Autodesk Inventor part; units mm, degrees
ref_plane "YZ Plane" through (0, 0, 0) normal (1, 0, 0) x (0, 1, 0)
ref_plane "XZ Plane" through (0, 0, 0) normal (0, 1, 0) x (-1, 0, 0)
ref_plane "XY Plane" through (0, 0, 0) normal (0, 0, 1) x (1, 0, 0)
sketch "Boceto1" plane through (0, 0, 0) normal (0, 1, 0) x (-1, 0, 0)
  circle A0 centre (0, 0) radius 19.6
  dimension "d0" = 39.2
extrude "Extrusión1" add sketch "Boceto1" along normal blind 60
sketch "Boceto2" plane through (0, 60, 0) normal (0, 1, 0) x (1, 0, 0)
  circle A0 centre (0, 0) radius 19.6
hole "Agujero1" at (0, 60, 0) direction (0, -1, 0) diameter 35 depth 20 tip angle 118
sketch "Boceto3" plane through (0, 0, 0) normal (0, -1, 0) x (1, 0, 0)
  circle A0 centre (0, 0) radius 19.6
hole "Agujero2" at (0, 0, 0) direction (0, 1, 0) diameter 10 depth 20 tip angle 118
thread "Rosca1"
fillet "Empalme1" radius 10 1 edges at (19.6, 0, 0)
properties part number "Casquillo"
Can you work these out from the model? Positions are in its coordinate system, mm. A direction names the side the tool comes from. Round coordinates to 2 decimals unless told otherwise and drop trailing zeros. Order: outer loops, then holes, each group sorted by start corner. A loop starts at its lowest first (then second) coordinate and runs counter-clockwise, first axis right, second up. Notation, with made-up numbers: M 87,-34 L 99,-34 A27 ccw 99,-14 Z; hole C 89,62 d11. An arc over 180 degrees is marked long. Use a Markdown table: item, result.
1) Imagine slicing it at A-A (y = 37.5). List the corners of the cut face in (x, z) for me, then the cut area to 3 significant figures.
Geometry says:
| item | result |
|---|---|
| outline | C 0,0 d39.2; hole C 0,0 d26.68 |
| area | 648 mm² |
2) I'm going to push flat-ended pins straight in: P1, Ø5, axis at y = 30.5, z = 4, coming from the +X side; P2, Ø1.5, axis at y = 17.5, z = -3.5, coming from the -X side; P3, Ø2, axis at y = 17, z = 12.5, coming from the -X side. Where does each tip first touch, or does it pass through?
Geometry says:
| item | result |
|---|---|
| P1 | stops at x = 19.54 |
| P2 | stops at x = -19.41 |
| P3 | stops at x = -15.87 |
3) On a 3-axis mill with a long thin cutter (end or side, diameter ignored), from which of +Z, -Z, +X, -X, +Y, -Y can I reach the whole of each face in a straight line? I mean faces 1 (the face through (-4, 0, -4)), 2 (the face through (4.88, 10.14, 1.08)). Say none if no direction works.
Geometry says:
| item | result |
|---|---|
| face 1 | +Z, -Z, +X, -X, -Y |
| face 2 | -Y |
4) If we mould it in two halves opening along Z, with no side actions, what happens to faces 3 (the face through (7.4, 60, 16.1)), 4 (the face through (4.249, 34.65, 19.134)), 5 (the face through (10.648, 49.86, -13.887))? For each: +Z half, -Z half, draft (parallel to the pull), parting line (faces both ways), or undercut.
Geometry says:
| item | result |
|---|---|
| face 3 | draft |
| face 4 | parting line |
| face 5 | undercut |
5) Imagine slicing it at B-B (y = 31). List the corners of the cut face in (x, z) for me, then the cut area to 3 significant figures.
Geometry says:
| item | result |
|---|---|
| outline | C 0,0 d39.2; hole C 0,0 d5.04 |
| area | 1,190 mm² |
6) If I drill on line 1 along Z through (x, y) = (0, 12); line 2 along Z through (x, y) = (0, 48); line 3 along X through (y, z) = (55, -3.5), over which ranges is the centre line in solid material (lowest first)?
Geometry says:
| item | result |
|---|---|
| line 1 | z = -19.6 to -5, 5 to 19.6 |
| line 2 | z = -19.6 to -17.5, 17.5 to 19.6 |
| line 3 | x = -19.28 to -17.15, 17.15 to 19.28 |
